For this review, take the finished solid that the model builds, in its own axes (mm). Coordinates: 2 decimals unless noted, no trailing zeros. Write each loop counter-clockwise with the first axis right and the second up, starting at its lowest first coordinate (ties: lowest second). Pieces come first, ordered by that corner, then holes.
```python
from build123d import *

# Parameters (mm, degrees)
SKETCH1_R           = 1
BOSS_EXTRUDE1_DEPTH = 6


with BuildPart() as part:
    # Sketch1 → Boss-Extrude1 (new body)
    with BuildSketch(Plane(origin=(0, 0, 0), x_dir=(1, 0, 0), z_dir=(0, 1, 0))):
        with BuildLine():
            Line((30, -63.5), (0, -63.5))
            ThreePointArc((0, -63.5), (-2.474873734, -62.474873734), (-3.5, -60))
            Line((-3.5, -60), (-3.5, 0))
            ThreePointArc((-3.5, 0), (-0.804135222, 3.406371463), (3.130495168, 1.565247584))
            Line((3.130495168, 1.565247584), (33.130495168, -58.434752416))
            ThreePointArc((33.130495168, -58.434752416), (32.977277829, -61.840058892), (30, -63.5))
        make_face()
        with Locations(Location((0, 0, 0), (0, 0, 270))):
            Circle(SKETCH1_R, mode=Mode.SUBTRACT)
        with Locations(Location((30, -60, 0), (0, 0, 270))):
            Circle(SKETCH1_R, mode=Mode.SUBTRACT)
    extrude(amount=BOSS_EXTRUDE1_DEPTH)


solid = part.part
```
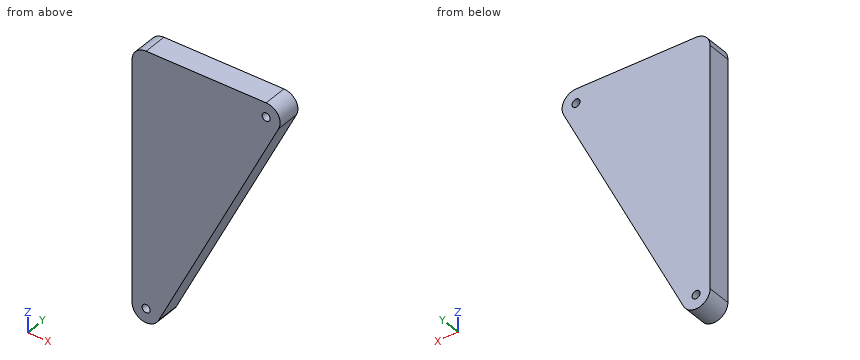
Q1. Add section B-B (z = 37). State the section outline as (x, y) points, then the cut area to 3 significant figures.
Ans:
outline: (-3.5, 0) - (22.41, 0) - (22.41, 6) - (-3.5, 6) - close
area: 155 mm2
Q2. Add section C-C (x = 24.5). State the section outline as (y, z) points.
Ans:
outline: (0, 41.17) - (6, 41.17) - (6, 63.5) - (0, 63.5) - close
Q3. Clearance check with flat-ended pins moving along their axes: pin 1 Ø2 at (x, y) = (25.5, 2.5) entering from -Z; pin 2 Ø6 at (x, z) = (28, 44) entering from +Y; pin 3 Ø3 at (y, z) = (2.5, 22.5) entering from +X. State where each tip first meets the part, or that it passes through.
Ans:
pin 1: stops at z = 41.17
pin 2: stops at y = 6
pin 3: stops at x = 15.91
Q4. Add section A-A (y = 4.3). State the section outline as (x, z) points, then the cut area to 3 significant figures.
Ans:
outline: (-3.5, 0) arc R3.5 ccw to (3.13, -1.57) - (33.13, 58.43) arc R3.5 ccw to (30, 63.5) - (0, 63.5) arc R3.5 ccw to (-3.5, 60) - close; hole circle Ø2 at (0, 0); hole circle Ø2 at (30, 60)
area: 1,480 mm2
Q5. For probe 1 along X at (y, z) = (4.3, 60); probe 2 along X at (y, z) = (4, 0); probe 3 along X at (y, z) = (1.3, 41.5), list the stretches that pass through material, from the lowest coordinate up.
Ans:
probe 1: x = -3.5 to 29, 31 to 33.5
probe 2: x = -3.5 to -1, 1 to 3.91
probe 3: x = -3.5 to 24.66
